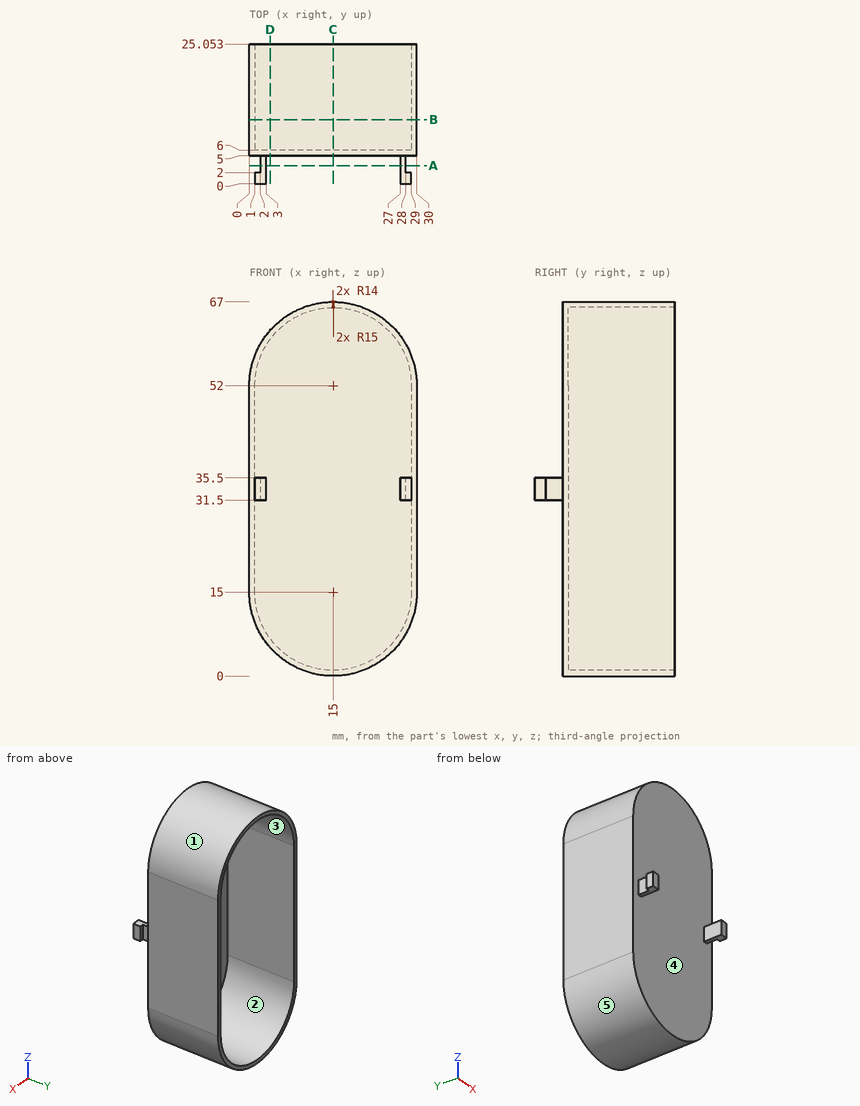
Source: three-view drawing plus pictorial views. Frame: mm from the lowest corner of the part. A direction names the side the tool comes from. Coordinates: 2 decimals unless noted, no trailing zeros. Write each loop counter-clockwise with the first axis right and the second up, starting at its lowest first coordinate (ties: lowest second). Pieces come first, ordered by that corner, then holes. Notation, with made-up numbers: (24, 23) - (69, 23) arc R21 cw to (69, 29) - close; hole circle Ø6 at (-32, 45). An arc over 180 degrees is marked (long way). Answer as a JSON object with one key per item and string values.
Q1. Section query B-B, the plane y = 11.5. Output: boundary loops of the cut face in (x, z), plus the area to 3 significant figures.
Ans:
{"outline": "(0, 15) arc R15 ccw to (30, 15) - (30, 52) arc R15 ccw to (0, 52) - close; hole (1, 15) arc R14 ccw to (29, 15) - (29, 52) arc R14 ccw to (1, 52) - close", "area": "165 mm2"}
Q2. Section query C-C, the plane x = 15. Output: boundary loops of the cut face in (y, z), plus the area to 3 significant figures.
Ans:
{"outline": "(5, 0) - (25.05, 0) - (25.05, 1) - (6, 1) - (6, 66) - (25.05, 66) - (25.05, 67) - (5, 67) - close", "area": "105 mm2"}
Q3. Material intervals for line 1 (X direction, y = 18.75, z = 50); line 2 (Y direction, x = 20, z = 5.5); line 3 (Y direction, x = 25, z = 63), sorted ascending. Write a range as [from, to].
Ans:
{"line 1": "x = [0, 1], [29, 30]", "line 2": "y = [5, 6]", "line 3": "y = [5, 25.05]"}
Q4. Set-up query: the marked faces 1 and 2. Return all of +Z, -Z, +X, -X, +Y, -Y with unobstructed straight access to the full face (end or side cutting, diameter ignored); none if empty.
Ans:
{"face 1": "+Z, +Y, -Y", "face 2": "+Y"}
Q5. Section query D-D, the plane x = 3.75. Output: boundary loops of the cut face in (y, z), plus the area to 3 significant figures.
Ans:
{"outline": "(5, 5.08) - (25.05, 5.08) - (25.05, 6.67) - (6, 6.67) - (6, 60.33) - (25.05, 60.33) - (25.05, 61.92) - (5, 61.92) - close", "area": "117 mm2"}
Q6. Section query A-A, the plane y = 3.25. Output: boundary loops of the cut face in (x, z).
Ans:
{"outline": "(2, 31.5) - (3, 31.5) - (3, 35.5) - (2, 35.5) - close; (27, 31.5) - (28, 31.5) - (28, 35.5) - (27, 35.5) - close"}
Q7. First-contact query: pin 1 Ø2 at (y, z) = (0.5, 33.5) entering from -X; pin 2 Ø1 at (y, z) = (10, 9.5) entering from -X; pin 3 Ø1.5 at (x, y) = (14, 12) entering from -Z; pin 4 Ø0.6 at (x, y) = (28.5, 3) entering from -Z. Flat tips, straight axial feed; report the tip coordinate or a pass-through.
Ans:
{"pin 1": "stops at x = 1", "pin 2": "stops at x = 0.86", "pin 3": "stops at z = 0", "pin 4": "passes through"}
Q8. Draft query along Z for the marked faces 3, 4 and 5. Return one class per face: released by +Z, released by -Z, zero draft, split by the parting line, or undercut.
Ans:
{"face 3": "undercut", "face 4": "zero draft", "face 5": "released by -Z"}
